The figure shows three views and two pictorial views of one solid part (mm, origin at its lowest corner). Answer the questions. Round coordinates to 2 decimals unless told otherwise and drop trailing zeros. Order: outer loops, then holes, each group sorted by start corner. A loop starts at its lowest first (then second) coordinate and runs counter-clockwise, first axis right, second up. Notation, with made-up numbers: (61, 37.25) - (114, 37.25) arc R5 cw to (114, 45.25) - close; hole circle Ø2 at (80, -10). An arc over 180 degrees is marked (long way). Write item = value, one per line.
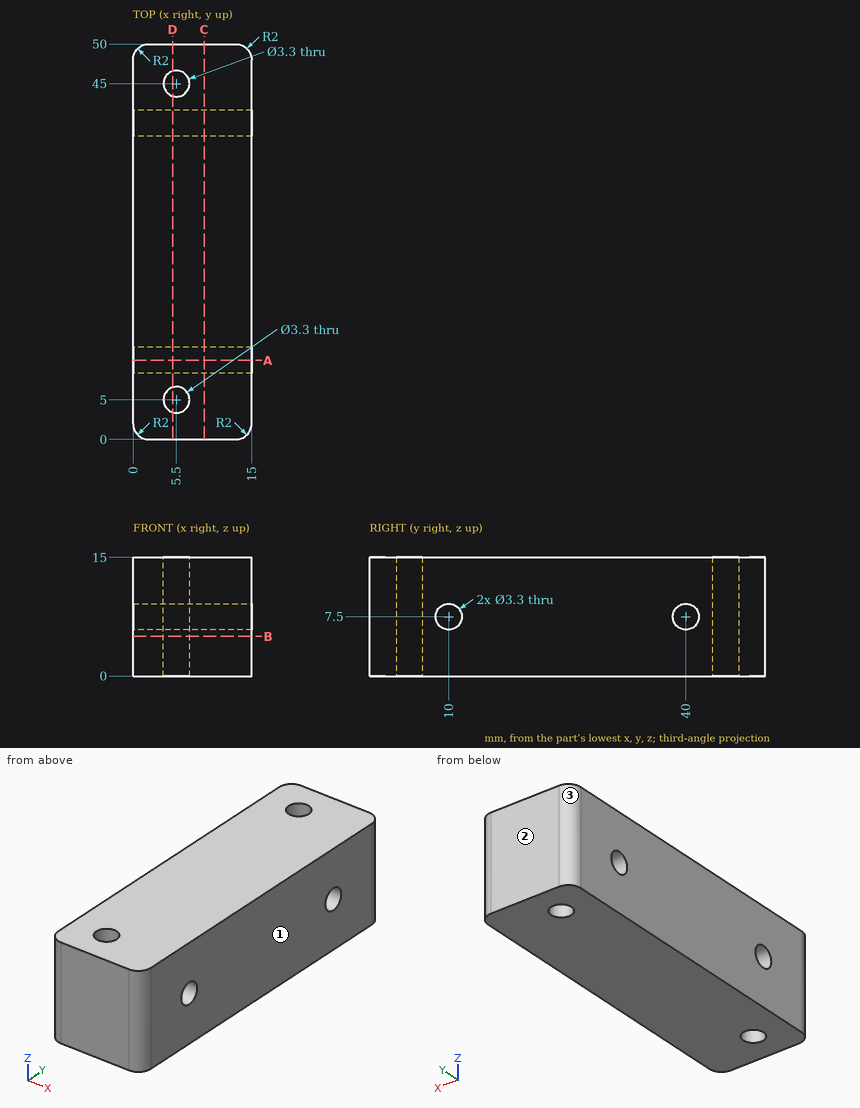
Q1. Find the intervals of material crossed by line 1 (Y direction, x = 10.25, z = 7.5); line 2 (Y direction, x = 10, z = 8.75); line 3 (X direction, y = 45, z = 9.25), in increasing order. Write a range as from..to.
Model answer:
line_1 = 0..8.35, 11.65..38.35, 41.65..50
line_2 = 0..8.92, 11.08..38.92, 41.08..50
line_3 = 0..3.85, 7.15..15
Q2. Determine the mould class of the marked faces 1, 2 and 3 for opening direction X: released by +X, released by -X, zero draft, split by the parting line, or undercut.
Model answer:
face_1 = released by +X
face_2 = zero draft
face_3 = released by -X
Q3. A flat-ended cylindrical pin translates along its axis: P1, Ø5, axis at x = 3.5, z = 2, coming from the -Y side. Find the tip coordinate at first contact, or state that the pin passes through.
Model answer:
P1 = 0
Q4. Section C-C on x = 9 is taken. Determine the outline of the cut face in (y, z).
Model answer:
outline = (0, 0) - (50, 0) - (50, 15) - (0, 15) - close; hole circle Ø3.3 at (10, 7.5); hole circle Ø3.3 at (40, 7.5)
Q5. Section D-D on x = 5 is taken. Determine the outline of the cut face in (y, z).
Model answer:
outline = (0, 0) - (3.43, 0) - (3.43, 15) - (0, 15) - close; (6.57, 0) - (43.43, 0) - (43.43, 15) - (6.57, 15) - close; (46.57, 0) - (50, 0) - (50, 15) - (46.57, 15) - close; hole circle Ø3.3 at (10, 7.5); hole circle Ø3.3 at (40, 7.5)
Q6. Section B-B on z = 5 is taken. Determine the outline of the cut face in (x, y).
Model answer:
outline = (0, 2) arc R2 ccw to (2, 0) - (13, 0) arc R2 ccw to (15, 2) - (15, 48) arc R2 ccw to (13, 50) - (2, 50) arc R2 ccw to (0, 48) - close; hole circle Ø3.3 at (5.5, 5); hole circle Ø3.3 at (5.5, 45)
Q7. Section A-A on y = 10 is taken. Determine the outline of the cut face in (x, z), then the cut area to 4 significant figures.
Model answer:
outline = (0, 0) - (15, 0) - (15, 5.85) - (0, 5.85) - close; (0, 9.15) - (15, 9.15) - (15, 15) - (0, 15) - close
area = 175.5 mm^2
